from build123d import *

# Parameters (mm, degrees)
SKETCH_1_W                            = 23
SKETCH_1_H                            = 12
SG90_CASE_PHOTO_APPROX23X12X22_DEPTH  = 22
SG90_EARS_APPROX32_START              = 16
SKETCH_2_W                            = 32
SKETCH_2_H                            = 12
SG90_EARS_APPROX32_DEPTH              = 2
SKETCH_3_R                            = 5.5
SG90_TOP_BOSS_APPROX_DEPTH            = 26
SKETCH_4_R                            = 2.4
SG90_SHAFT_ENVELOPE_NO_SPLINE_DEPTH   = 29
SG90_EAR_HOLES_REFERENCE28_DEPTH      = 34.660065359
SG90_EAR_HOLES_REFERENCE28_DEPTH_BACK = 34.660065359
SKETCH_5_R                            = 1.1


with BuildPart() as part:
    # 草图1 → SG90_case_PHOTO_APPROX23x12x22 (new body)
    with BuildSketch(Plane.XY):
        Rectangle(SKETCH_1_W, SKETCH_1_H)
    extrude(amount=SG90_CASE_PHOTO_APPROX23X12X22_DEPTH)

    # 草图2 → SG90_ears_APPROX32 (add)
    with BuildSketch(Plane.XY.offset(SG90_EARS_APPROX32_START)):
        Rectangle(SKETCH_2_W, SKETCH_2_H)
    extrude(amount=SG90_EARS_APPROX32_DEPTH)

    # 草图3 → SG90_top_boss_APPROX (add)
    with BuildSketch(Plane.XY):
        with Locations(Location((-5.5, 0, 0), (0, 0, 180))):
            Circle(SKETCH_3_R)
    extrude(amount=SG90_TOP_BOSS_APPROX_DEPTH)

    # 草图4 → SG90_shaft_envelope_NO_SPLINE (add)
    with BuildSketch(Plane.XY):
        with Locations(Location((-5.5, 0, 0), (0, 0, 180))):
            Circle(SKETCH_4_R)
    extrude(amount=SG90_SHAFT_ENVELOPE_NO_SPLINE_DEPTH)

    # 草图5 → SG90_ear_holes_REFERENCE28 (cut, two sides: drawn at the far end of the back side and taken through both)
    with BuildSketch(Plane.XY.offset(-SG90_EAR_HOLES_REFERENCE28_DEPTH_BACK)):
        with Locations((-14, 0)):
            Circle(SKETCH_5_R)
        with Locations((14, 0)):
            Circle(SKETCH_5_R)
    extrude(amount=SG90_EAR_HOLES_REFERENCE28_DEPTH + SG90_EAR_HOLES_REFERENCE28_DEPTH_BACK, mode=Mode.SUBTRACT)


solid = part.part
Work out the finished part from the listing and answer in its coordinate system (mm). A direction names the side the tool comes from. Give positions to 0.01 mm unless a question says otherwise; leave off trailing zeros. Loops run counter-clockwise (first coordinate to the right, second up) from the corner with the lowest first, then second, coordinate; pieces in that order, holes last. Notation, with made-up numbers: (0, 60.5) -> (54, 60.5) arc R18 cw to (54, 91.5) -> close; hole circle Ø6 at (-24, 86.5). An arc over 180 degrees is marked (long way). Use a Markdown table: item, result. Add a question column.
1. For faces 1 (the flat face through (-13.8, 1.4, 16)), 2 (the flat face through (2, 0, 22)), 3 (the flat face through (12.7, 0.1, 16)), 4 (the flat face through (12.7, 0.1, 18)), 5 (the flat face through (-11.5, 0, 20)), determine the directions among +Z, -Z, +X, -X, +Y, -Y from which every point of the face is accessible in a straight line to the end or side of a thin tool.
2. Flat-ended cylindrical pins translate along their axes: pin 1 Ø2 at (y, z) = (-2.5, 21) entering from -X; pin 2 Ø2 at (x, y) = (-14.5, 1.5) entering from +Z; pin 3 Ø6 at (y, z) = (2, 7.5) entering from +X; pin 4 Ø4 at (x, y) = (-0.5, 0) entering from -Z. Find the tip coordinate at first contact, or state that the pin passes through.
3. Find the intervals of material crossed by probe 1 along X at (y, z) = (0, 17.55); probe 2 along Y at (x, z) = (-14, 17); probe 3 along X at (y, z) = (-1.5, 11), in increasing order.
4. Section A-A on y = 0 is taken. Determine the outline of the cut face in (x, z).
5. Section C-C on x = -5.5 is taken. Determine the outline of the cut face in (y, z).
6. Determine the mould class of faces 6 (the cylindrical face through (12.9, 0, 17)), 7 (the flat face through (11.5, 0, 8)), 8 (the cylindrical face through (-8, 4.9, 24)) for opening direction Y: released by +Y, released by -Y, zero draft, split by the parting line, or undercut.
7. Section D-D on y = -4.5 is taken. Determine the outline of the cut face in (x, z).
8. Section B-B on x = -14 is taken. Determine the outline of the cut face in (y, z), and give its area (3 significant figures).
Results below:
| question | item | result |
|---|---|---|
| 1 | face 1 | -Z, -X, +Y, -Y |
| 1 | face 2 | +Z |
| 1 | face 3 | -Z, +X, +Y, -Y |
| 1 | face 4 | +Z, +X, +Y, -Y |
| 1 | face 5 | +Z, -X, +Y, -Y |
| 2 | pin 1 | stops at x = -11.5 |
| 2 | pin 2 | stops at z = 18 |
| 2 | pin 3 | stops at x = 11.5 |
| 2 | pin 4 | stops at z = 0 |
| 3 | probe 1 | x = -16 to -15.1, -12.9 to 12.9, 15.1 to 16 |
| 3 | probe 2 | y = -6 to -1.1, 1.1 to 6 |
| 3 | probe 3 | x = -11.5 to 11.5 |
| 4 | outline | (-16, 16) -> (-15.1, 16) -> (-15.1, 18) -> (-16, 18) -> close; (-12.9, 16) -> (-11.5, 16) -> (-11.5, 0) -> (11.5, 0) -> (11.5, 16) -> (12.9, 16) -> (12.9, 18) -> (11.5, 18) -> (11.5, 22) -> (0, 22) -> (0, 26) -> (-3.1, 26) -> (-3.1, 29) -> (-7.9, 29) -> (-7.9, 26) -> (-11, 26) -> (-11, 22) -> (-11.5, 22) -> (-11.5, 18) -> (-12.9, 18) -> close; (15.1, 16) -> (16, 16) -> (16, 18) -> (15.1, 18) -> close |
| 5 | outline | (-6, 0) -> (6, 0) -> (6, 22) -> (5.5, 22) -> (5.5, 26) -> (2.4, 26) -> (2.4, 29) -> (-2.4, 29) -> (-2.4, 26) -> (-5.5, 26) -> (-5.5, 22) -> (-6, 22) -> close |
| 6 | face 6 | undercut |
| 6 | face 7 | zero draft |
| 6 | face 8 | split by the parting line |
| 7 | outline | (-16, 16) -> (-11.5, 16) -> (-11.5, 0) -> (11.5, 0) -> (11.5, 16) -> (16, 16) -> (16, 18) -> (11.5, 18) -> (11.5, 22) -> (-2.34, 22) -> (-2.34, 26) -> (-8.66, 26) -> (-8.66, 22) -> (-11.5, 22) -> (-11.5, 18) -> (-16, 18) -> close |
| 8 | outline | (-6, 16) -> (-1.1, 16) -> (-1.1, 18) -> (-6, 18) -> close; (1.1, 16) -> (6, 16) -> (6, 18) -> (1.1, 18) -> close |
| 8 | area | 19.6 mm^2 |
